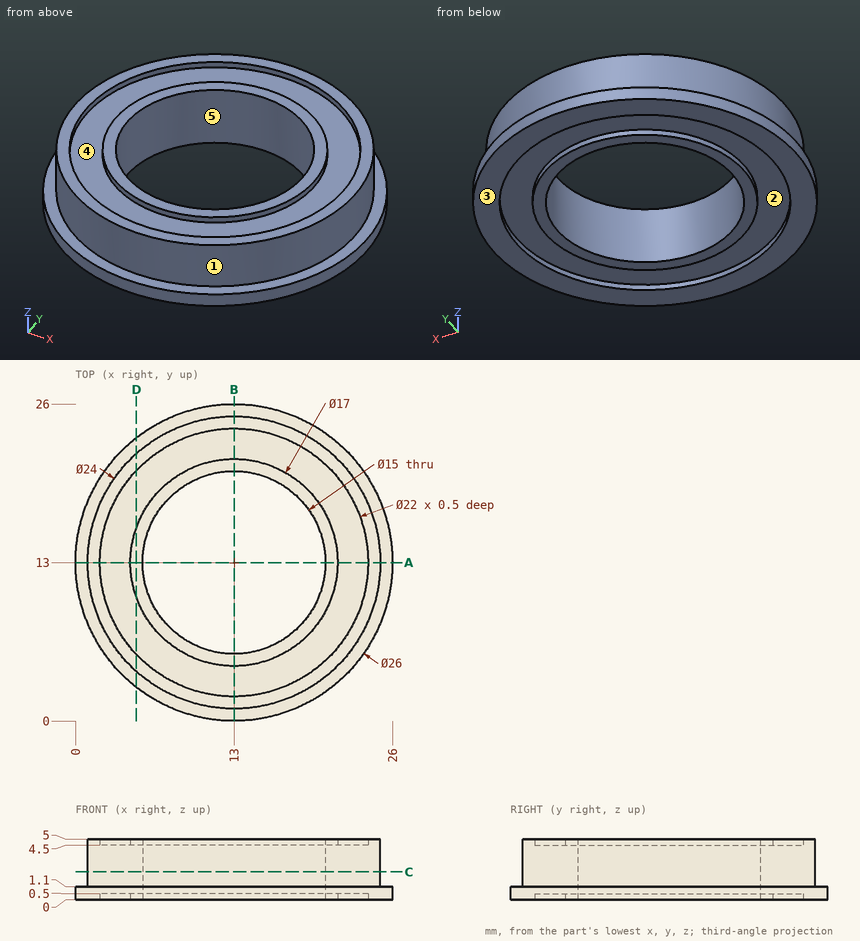
Could you check a few things on this drawing? It's one solid part, dimensions in mm from its lowest x, y, z. A direction names the side the tool comes from. Coordinates: 2 decimals unless noted, no trailing zeros. Loops run counter-clockwise (first coordinate to the right, second up) from the corner with the lowest first, then second, coordinate; pieces in that order, holes last.
1. For P1, Ø2, axis at y = 18.5, z = 3, coming from the -X side; P2, Ø2, axis at x = 5.5, z = 3, coming from the -Y side, each with a flat end and sliding along its axis, tell me the tip position at first contact or that it passes through.
2. Imagine slicing it at D-D (x = 5). Please give me the cut outline in (y, z).
3. I need wall thicknesses on L1, parallel to Y at x = 13, z = 4.75; L2, parallel to Y at x = 13, z = 0.45; L3, parallel to Y at x = 13, z = 3.5. Which ranges of each line are inside material? Lowest first, please.
4. We'd pull the mould along Y, two halves only. Please class the marked faces 1, 2 and 3: released by +Y, released by -Y, zero draft, split by the parting line, or undercut.
5. Imagine slicing it at A-A (y = 13). Please give me the cut outline in (x, z).
6. Imagine slicing it at C-C (z = 2.3). Please give me the cut outline in (x, y).
7. For the marked faces 4 and 5, which set-ups out of +Z, -Z, +X, -X, +Y, -Y let a thin tool reach every point of the face, with its end or its side?
Computed values:
1. P1: stops at x = 1.88
1. P2: stops at y = 2.91
2. outline: (2.75, 0) - (5.45, 0) - (5.45, 0.5) - (10.13, 0.5) - (10.13, 0) - (15.87, 0) - (15.87, 0.5) - (20.55, 0.5) - (20.55, 0) - (23.25, 0) - (23.25, 1.1) - (21.94, 1.1) - (21.94, 5) - (20.55, 5) - (20.55, 4.5) - (15.87, 4.5) - (15.87, 5) - (10.13, 5) - (10.13, 4.5) - (5.45, 4.5) - (5.45, 5) - (4.06, 5) - (4.06, 1.1) - (2.75, 1.1) - close
3. L1: y = 1 to 2, 4.5 to 5.5, 20.5 to 21.5, 24 to 25
3. L2: y = 0 to 2, 4.5 to 5.5, 20.5 to 21.5, 24 to 26
3. L3: y = 1 to 5.5, 20.5 to 25
4. face 1: split by the parting line
4. face 2: undercut
4. face 3: zero draft
5. outline: (0, 0) - (2, 0) - (2, 0.5) - (4.5, 0.5) - (4.5, 0) - (5.5, 0) - (5.5, 5) - (4.5, 5) - (4.5, 4.5) - (2, 4.5) - (2, 5) - (1, 5) - (1, 1.1) - (0, 1.1) - close; (20.5, 0) - (21.5, 0) - (21.5, 0.5) - (24, 0.5) - (24, 0) - (26, 0) - (26, 1.1) - (25, 1.1) - (25, 5) - (24, 5) - (24, 4.5) - (21.5, 4.5) - (21.5, 5) - (20.5, 5) - close
6. outline: circle Ø24 at (13, 13); hole circle Ø15 at (13, 13)
7. face 4: +Z
7. face 5: +Z, -Z
